CAD build for the part. Positions are in the model's coordinates, mm. A direction names the side the tool comes from. Coordinates: 2 decimals unless noted, no trailing zeros. Loops run counter-clockwise (first coordinate to the right, second up) from the corner with the lowest first, then second, coordinate; pieces in that order, holes last. Notation, with made-up numbers: (8, 10) - (49, 10) arc R34 ccw to (49, 49) - close; hole circle Ø9 at (47.25, -25). An arc over 180 degrees is marked (long way). Put each result on its own line as item: value.
```python
from build123d import *

# Parameters (mm, degrees)
SKETCH_1_R          = 1.569016128
EXTRUDE_1_DEPTH     = 2
FILLET_1_R          = 10
CUT_EXTRUDE_1_DEPTH = 2


with BuildPart() as part:
    # 草图1 → 凸台-拉伸1 (new body)
    with BuildSketch(Plane(origin=(0, 0, 0), x_dir=(1, 0, 0), z_dir=(0, 1, 0))):
        Polygon((-52.5, 70), (-40, 57.5), (40, 57.5), (52.5, 70), (70, 70), (70, 52.5), (57.5, 40), (57.5, -40), (70, -52.5), (70, -70), (52.5, -70), (40, -57.5), (-40, -57.5), (-52.5, -70), (-70, -70), (-70, -52.5), (-57.5, -40), (-57.5, 40), (-70, 52.5), (-70, 70), align=None)
        with Locations(Location((-63.74128019, 63.74128019, 0), (0, 0, 270))):
            Circle(SKETCH_1_R, mode=Mode.SUBTRACT)
        with Locations(Location((63.74128019, 63.74128019, 0), (0, 0, 270))):
            Circle(SKETCH_1_R, mode=Mode.SUBTRACT)
        with Locations(Location((63.74128019, -63.74128019, 0), (0, 0, 270))):
            Circle(SKETCH_1_R, mode=Mode.SUBTRACT)
        with Locations(Location((-63.74128019, -63.74128019, 0), (0, 0, 270))):
            Circle(SKETCH_1_R, mode=Mode.SUBTRACT)
    extrude(amount=EXTRUDE_1_DEPTH)

    # 圆角1
    fillet_1_edges = [part.edges().sort_by_distance(p)[0] for p in [
        (57.5, 1, -40),
        (57.5, 1, 40),
        (40, 1, 57.5),
        (-40, 1, 57.5),
        (-57.5, 1, 40),
        (-57.5, 1, -40),
        (-40, 1, -57.5),
        (40, 1, -57.5),
    ]]
    fillet(fillet_1_edges, radius=FILLET_1_R)

    # 草图2 → 切除-拉伸1 (cut)
    with BuildSketch(Plane(origin=(0, 2, 0), x_dir=(1, 0, 0), z_dir=(0, 1, 0))):
        with BuildLine():
            Line((-5, -40), (-5, 40))
            ThreePointArc((-5, 40), (0, 45), (5, 40))
            Line((5, 40), (5, -40))
            ThreePointArc((5, -40), (0, -45), (-5, -40))
        make_face()
        with BuildLine():
            Line((11, -40), (11, 40))
            ThreePointArc((11, 40), (16, 45), (21, 40))
            Line((21, 40), (21, -40))
            ThreePointArc((21, -40), (16, -45), (11, -40))
        make_face()
        with BuildLine():
            Line((27, -40), (27, 40))
            ThreePointArc((27, 40), (32, 45), (37, 40))
            Line((37, 40), (37, -40))
            ThreePointArc((37, -40), (32, -45), (27, -40))
        make_face()
        with BuildLine():
            Line((-21, -40), (-21, 40))
            ThreePointArc((-21, 40), (-16, 45), (-11, 40))
            Line((-11, 40), (-11, -40))
            ThreePointArc((-11, -40), (-16, -45), (-21, -40))
        make_face()
        with BuildLine():
            Line((-37, -40), (-37, 40))
            ThreePointArc((-37, 40), (-32, 45), (-27, 40))
            Line((-27, 40), (-27, -40))
            ThreePointArc((-27, -40), (-32, -45), (-37, -40))
        make_face()
    extrude(amount=-CUT_EXTRUDE_1_DEPTH, mode=Mode.SUBTRACT)


solid = part.part
```
Q1. Mould opens along Z. For faces 5 (the flat face through (-65.1, 1, -47.6)), 6 (the flat face through (1, 2, 46)), 7 (the flat face through (47.8, 1, 65.3)) say: +Z half, -Z half, draft (parallel to the pull), parting line (faces both ways), or undercut.
Determined:
face 5: undercut
face 6: draft
face 7: +Z half
Q2. Slice it at C-C, the plane y = 0.7. State how many separate pieces and enclosed holes the cut face has, then the cut area to 3 significant figures.
Determined:
separate pieces: 1
enclosed holes: 9
area: 10,600 mm2
Q3. Tool access for faces 1 (the flat face through (47.6, 1, -65.1)), 2 (the cylindrical face through (16, 1, -45)), 3 (the flat face through (-65.3, 1, 47.8)), 4 (the flat face through (65.3, 1, -47.8)): list every direction of +Z, -Z, +X, -X, +Y, -Y with a clear straight run to the whole face (end or side of a thin tool).
Determined:
face 1: -Z, +Y, -Y
face 2: +Y, -Y
face 3: -X, +Y, -Y
face 4: +X, +Y, -Y
Q4. Slice it at A-A, the plane z = -19. Give the cut face in (x, y), then the cut area to 3 significant figures.
Determined:
outline: (-57.5, 0) - (-37, 0) - (-37, 2) - (-57.5, 2) - close; (-27, 0) - (-21, 0) - (-21, 2) - (-27, 2) - close; (-11, 0) - (-5, 0) - (-5, 2) - (-11, 2) - close; (5, 0) - (11, 0) - (11, 2) - (5, 2) - close; (21, 0) - (27, 0) - (27, 2) - (21, 2) - close; (37, 0) - (57.5, 0) - (57.5, 2) - (37, 2) - close
area: 130 mm2
Q5. Slice it at B-B, the plane x = -16. Give the cut face in (y, z).
Determined:
outline: (0, -57.5) - (2, -57.5) - (2, -45) - (0, -45) - close; (0, 45) - (2, 45) - (2, 57.5) - (0, 57.5) - close
Q6. Slice it at D-D, the plane x = -41. Give the cut face in (y, z), then the cut area to 3 significant figures.
Determined:
outline: (0, -58.92) - (2, -58.92) - (2, 58.92) - (0, 58.92) - close
area: 236 mm2
Q7. Pin check, flat tips, straight feed: pin 1 Ø0.6 at (y, z) = (0.5, -17.5) entering from -X; pin 2 Ø1 at (y, z) = (1, 19) entering from +X; pin 3 Ø1 at (x, y) = (-13, 1.5) entering from -Z. Stop position of each tip, or through.
Determined:
pin 1: x = -57.5
pin 2: x = 57.5
pin 3: z = -57.5
Q8. Wall check: L1, parallel to X at y = 1.5, z = 22.5; L2, parallel to Z at x = 32, y = 0.5; L3, parallel to X at y = 1, z = 43. Give the ranges that are in metal, low to high. Write a range as from..to.
Determined:
L1: -57.5..-37, -27..-21, -11..-5, 5..11, 21..27, 37..57.5
L2: -57.5..-45, 45..57.5
L3: -60.5..-36, -28..-20, -12..-4, 4..12, 20..28, 36..60.5
